Read the model definition and answer for the solid it produces. Units are mm, in the model's axes. A direction names the side the tool comes from. Coordinates: 2 decimals unless noted, no trailing zeros. Write each loop counter-clockwise with the first axis right and the second up, starting at its lowest first coordinate (ties: lowest second). Pieces come first, ordered by that corner, then holes.
Item 1: A tool of negligible diameter and unlimited length cuts with its end or side. For faces 1 (the face through (1, 10, 32)), 2 (the face through (26.68, 151.59, 6.93)), 3 (the face through (1, 5, 50)), from which of +Z, -Z, +X, -X, +Y, -Y can it reach the whole face along a straight path? Write none if from no direction.
Item 2: Section C-C (x = 27) is taken. Give the vertices of the cut face in (y, z), then the cut area to 3 significant figures.
Item 3: Determine the mould class of faces 4 (the face through (1, 86, 15)), 5 (the face through (14, 150, 8)), 6 (the face through (-39, 61, 14)) for opening direction Z: released by +Z, released by -Z, zero draft, split by the parting line, or undercut.
Item 4: Each of these flat-tipped pins is pushed along its axis until it touches: P1, Ø1, axis at x = 7.5, z = 40.5, coming from the +Y side; P2, Ø2.5, axis at y = 17, z = 8, coming from the +X side; P3, Ø8, axis at x = 6, y = 58.5, coming from the +Z side; P4, Ø0.9, axis at y = 151, z = 7, coming from the +X side. Where does it stop, or does it pass through?
Item 5: Straight lines are drawn through the part: probe 1 along Z at (x, y) = (-1, 60); probe 2 along Y at (x, z) = (23, 7); probe 3 along Z at (x, y) = (19, 108.5). For each, find the intervals that lie inside material, in ascending order.
Item 6: Section A-A (y = 60) is taken. Give the vertices of the cut face in (x, z), then the cut area to 3 significant figures.
Item 7: Section D-D (x = -27.5) is taken. Give the vertices of the cut face in (y, z).
Item 8: Section B-B (z = 7.5) is taken. Give the vertices of the cut face in (x, y), then the cut area to 3 significant figures.
from build123d import *

# Parameters (mm, degrees)
F1_DEPTH = 39
F2_R     = 5.5
F3_DEPTH = 100
F4_R     = 1.5
F5_DEPTH = 25


with BuildPart() as f1:
    # F0 (on Right) → F1 (new body, symmetric)
    with BuildSketch(Plane.YZ):
        Polygon((0, 50), (0, 0), (160, 0), (160, 15), (10, 15), (10, 50), align=None)
    extrude(amount=F1_DEPTH, both=True)

    # F2 (on face) → F3 (cut)
    with BuildSketch(Plane.YZ.offset(39)):
        with Locations((60, 7.5)):
            Circle(F2_R)
    extrude(amount=-F3_DEPTH, mode=Mode.SUBTRACT)

    # F4 (on face) → F5 (cut)
    with BuildSketch(Plane.YZ.offset(39)):
        with Locations((150.202468, 7.5)):
            Circle(F4_R)
        with Locations((16.434773, 7.5)):
            Circle(F4_R)
    extrude(amount=-F5_DEPTH, mode=Mode.SUBTRACT)


solid = f1.part
Established:
1. face 1: +Z, +X, -X, +Y
1. face 2: +X
1. face 3: +Z, +X, -X, +Y, -Y
2. outline: (0, 0) - (160, 0) - (160, 15) - (10, 15) - (10, 50) - (0, 50) - close; hole circle Ø3 at (16.43, 7.5); hole circle Ø11 at (60, 7.5); hole circle Ø3 at (150.2, 7.5)
2. area: 2,640 mm2
3. face 4: released by +Z
3. face 5: undercut
3. face 6: zero draft
4. P1: stops at y = 10
4. P2: stops at x = 39
4. P3: stops at z = 15
4. P4: stops at x = 14
5. probe 1: z = 0 to 2, 13 to 15
5. probe 2: y = 0 to 15.02, 17.85 to 54.52, 65.48 to 148.79, 151.62 to 160
5. probe 3: z = 0 to 15
6. outline: (-39, 0) - (39, 0) - (39, 2) - (-39, 2) - close; (-39, 13) - (39, 13) - (39, 15) - (-39, 15) - close
6. area: 312 mm2
7. outline: (0, 0) - (160, 0) - (160, 15) - (10, 15) - (10, 50) - (0, 50) - close; hole circle Ø11 at (60, 7.5)
8. outline: (-39, 0) - (39, 0) - (39, 14.93) - (14, 14.93) - (14, 17.93) - (39, 17.93) - (39, 54.5) - (-39, 54.5) - close; (-39, 65.5) - (39, 65.5) - (39, 148.7) - (14, 148.7) - (14, 151.7) - (39, 151.7) - (39, 160) - (-39, 160) - close
8. area: 11,500 mm2
